```python
from build123d import *

# Parameters (mm, degrees)
F1_DEPTH    = 63.5
F2_R        = 1.7934980513
F3_R        = 0.4788394015
F4_R        = 2.7306448225
F5_R        = 0.9937962324
F6_R        = 5.08
F7_R        = 1.519546052
F8_T1_DEPTH = 212.3191575165
F9_R        = 7.9959076321


# Not quite as in the source:
# - a fillet or chamfer that OpenCascade refuses, or shapes differently, is made with other operations: its cross-section is extruded or revolved along the edge and cut away or added


with BuildPart() as f1:
    # F0 (on Right) → F1 (new body)
    with BuildSketch(Plane.YZ):
        Polygon((-16.9031135738, 20.9204703569), (-26.4463126659, 0), (27.971111238, 0), (27.971111238, 20.9204703569), (-4.9152970314, 20.9204703569), (-7.6606271703, 14.2183713615), (-14.0469465405, 14.2183713615), (-11.3016164016, 20.9204703569), align=None)
    extrude(amount=F1_DEPTH)

    # F2
    f2_edges = [f1.edges().sort_by_distance(p)[0] for p in [
        (31.75, -4.915297, 20.92047),
    ]]
    fillet(f2_edges, radius=F2_R)

    # F3
    f3_edges = [f1.edges().sort_by_distance(p)[0] for p in [
        (31.75, -11.301616, 20.92047),
    ]]
    fillet(f3_edges, radius=F3_R)

    # F4
    f4_edges = [f1.edges().sort_by_distance(p)[0] for p in [
        (31.75, -7.660627, 14.218371),
    ]]
    fillet(f4_edges, radius=F4_R)

    # F5
    f5_edges = [f1.edges().sort_by_distance(p)[0] for p in [
        (31.75, -14.046947, 14.218371),
    ]]
    fillet(f5_edges, radius=F5_R)

    # F6
    f6_edges = [f1.edges().sort_by_distance(p)[0] for p in [
        (31.75, -16.903114, 20.92047),
    ]]
    fillet(f6_edges, radius=F6_R)

    # F7
    f7_edges = [f1.edges().sort_by_distance(p)[0] for p in [
        (31.75, -26.446313, 0),
    ]]
    fillet(f7_edges, radius=F7_R)

    # F8: fillet of radius 31.6329347077 on 1 edges, made by hand

    # F8_s2 → F8_t1 (cut)
    with BuildSketch(Plane.YZ.offset(-74.4095787583)):
        with BuildLine():
            ThreePointArc((27.971111238, 0), (16.3976050872, 15.1671535327), (-1.7927202653, 20.9204703569))
            Line((-1.7927202653, 20.9204703569), (27.971111238, 20.9204703569))
            Line((27.971111238, 20.9204703569), (27.971111238, 0))
        make_face()
    extrude(amount=F8_T1_DEPTH, mode=Mode.SUBTRACT)

    # F9
    f9_edges = [f1.edges().sort_by_distance(p)[0] for p in [
        (31.75, 27.971111, 0),
    ]]
    fillet(f9_edges, radius=F9_R)


solid = f1.part
```
Geometry: final body of the model. Coordinates: model frame, mm. A direction names the side the tool comes from. Coordinates: 2 decimals unless noted, no trailing zeros. Order: outer loops, then holes, each group sorted by start corner. A loop starts at its lowest first (then second) coordinate and runs counter-clockwise, first axis right, second up. Notation, with made-up numbers: (16.5, 3.25) -> (59.5, 3.25) arc R16 cw to (59.5, 18.25) -> close; hole circle Ø2 at (-28.75, -37.5). An arc over 180 degrees is marked (long way). Use CSV: the item, a comma, the result in double quotes.
1) Section B-B on y = 11. Output: boundary loops of the cut face in (x, z), then the cut area to 3 significant figures.
Findings:
outline,"(0, 0) -> (63.5, 0) -> (63.5, 18.22) -> (0, 18.22) -> close"
area,"1,160 mm^2"
2) Mould query, pull axis Z, two halves, no side actions, for faces 4 (the flat face through (31, -6, 0)), 5 (the cylindrical face through (32.194, 20.265, 5.546)), 6 (the cylindrical face through (32.19, -7.99, 14.67)), 7 (the flat face through (31, -11, 14.218)). Classes: +Z half, -Z half, draft (parallel to the pull), parting line (faces both ways), or undercut.
Findings:
face 4,"-Z half"
face 5,"parting line"
face 6,"+Z half"
face 7,"undercut"
3) Section C-C on z = 7.5. Output: boundary loops of the cut face in (x, y).
Findings:
outline,"(0, -23.03) -> (63.5, -23.03) -> (63.5, 20.63) -> (0, 20.63) -> close"
4) Pin query (flat end, axial travel): pin 1 Ø1.5 at (x, y) = (44.5, -20.5) entering from +Z; pin 2 Ø1 at (x, z) = (41.5, 12) entering from +Y; pin 3 Ø12 at (x, z) = (39, 11) entering from -Y. Return the tip coordinate at first contact, or that it passes through.
Findings:
pin 1,"stops at z = 14.68"
pin 2,"stops at y = 19.84"
pin 3,"stops at y = -24.17"
5) Access query for faces 1 (the cylindrical face through (32.194, -13.383, 14.647)), 2 (the flat face through (31.306, -6.158, 17.888)), 3 (the cylindrical face through (32.194, -16.35, 20.135)). Directions: +Z, -Z, +X, -X, +Y, -Y. A direction counts if a zero-diameter tool reaches every point of the face in a straight line with its end or side. Return the directions, or none.
Findings:
face 1,"+X, -X"
face 2,"+Z, +X, -X"
face 3,"+Z, +X, -X, -Y"
6) Line query: line 1 (Z direction, x = 6.5, y = -1.5); line 2 (Y direction, x = 11, z = 14.75); line 3 (Y direction, x = 14, z = 18.5). Output: solid intervals per line, ascending.
Findings:
line 1,"z = 0 to 20.92"
line 2,"y = -19.72 to -13.45, -7.87 to 16.98"
line 3,"y = -17.97 to -12.29, -5.91 to 10.34"
7) Section A-A on x = 40. Output: boundary loops of the cut face in (y, z).
Findings:
outline,"(-25.47, 2.15) arc R1.52 ccw to (-24.08, 0) -> (12.65, 0) arc R8 ccw to (17.54, 14.32) arc R31.63 ccw to (-1.79, 20.92) -> (-3.71, 20.92) arc R1.79 ccw to (-5.37, 19.81) -> (-6.97, 15.91) arc R2.73 cw to (-9.49, 14.22) -> (-12.57, 14.22) arc R0.99 cw to (-13.49, 15.59) -> (-11.57, 20.26) arc R0.48 ccw to (-12.02, 20.92) -> (-13.64, 20.92) arc R5.08 ccw to (-18.26, 17.95) -> close"
